Verification items for this drawing (mm, ordinates from the low corner). Coordinates: 2 decimals unless noted, no trailing zeros. Loops run counter-clockwise (first coordinate to the right, second up) from the corner with the lowest first, then second, coordinate; pieces in that order, holes last. Notation, with made-up numbers: M 36.5,27 L 40.5,27 A6 cw 40.5,35 Z; hole C -29,6.25 d4. An arc over 180 degrees is marked long. Write each question's results on one line, items separated by ' | '. Start each with the question number.
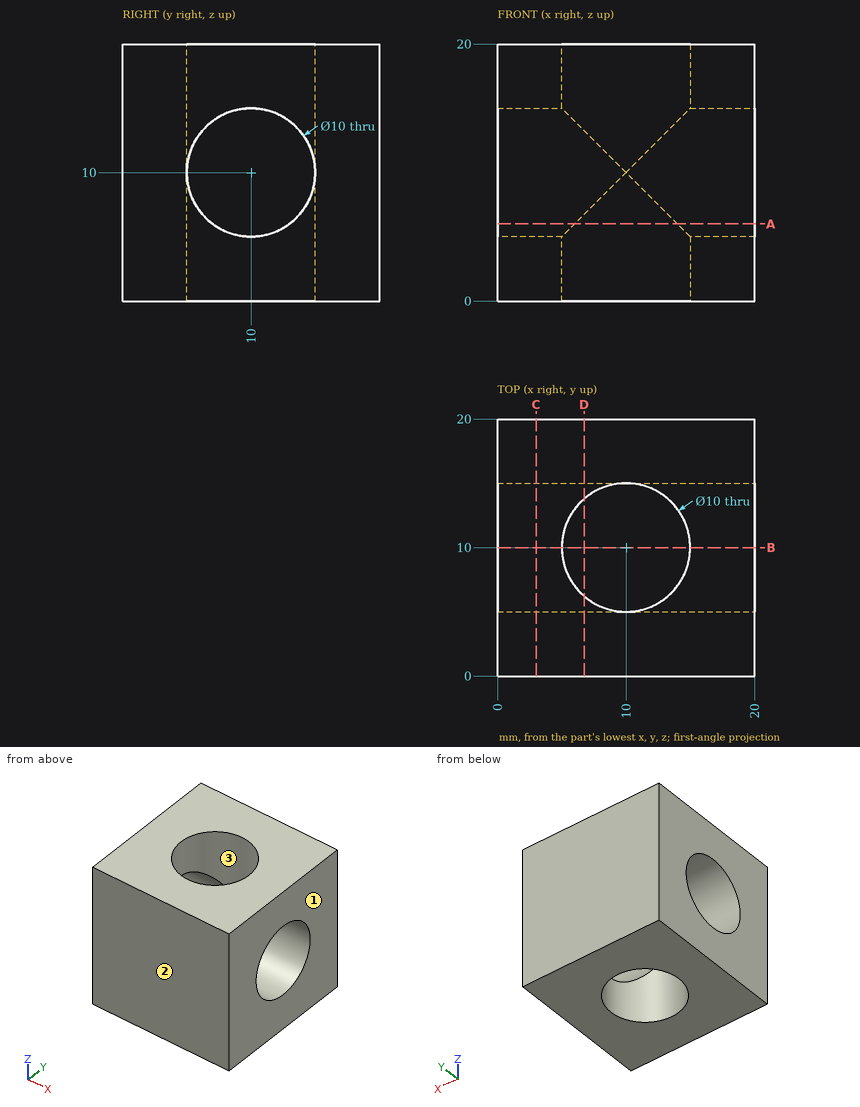
Item 1: Section check A-A (z = 6). Record the cut outline in (x, y).
Item 2: Release check for a two-part mould opening along X. For the marked faces 1, 2 and 3 record: +X half, -X half, draft (parallel to the pull), parting line (faces both ways), or undercut.
Item 3: Section check C-C (x = 3). Record the cut outline in (y, z).
Item 4: Depth check by flat-ended pin: P1, Ø10, axis at x = 13, z = 16.5, coming from the -Y side. Enter the tip coordinate at first touch or a pass-through.
Item 5: Section check D-D (x = 6.75). Record the cut outline in (y, z).
Item 6: Thickness scan on line 1 (Z direction, x = 4.5, y = 10). Record the ranges inside material, lowest first.
Item 7: Section check B-B (y = 10). Record the cut outline in (x, z), plus the area to 3 significant figures.
Computed values:
1) outline: M 0,0 L 20,0 L 20,7 L 14,7 A5 cw 6,7 L 0,7 Z; M 0,13 L 6,13 A5 cw 14,13 L 20,13 L 20,20 L 0,20 Z
2) face 1: +X half | face 2: draft | face 3: undercut
3) outline: M 0,0 L 20,0 L 20,20 L 0,20 Z; hole C 10,10 d10
4) P1: stops at y = 0
5) outline: M 0,0 L 6.2,0 L 6.2,6.75 A5 cw 6.2,13.25 L 6.2,20 L 0,20 Z; M 13.8,0 L 20,0 L 20,20 L 13.8,20 L 13.8,13.25 A5 cw 13.8,6.75 Z
6) line 1: z = 0 to 5, 15 to 20
7) outline: M 0,0 L 5,0 L 5,5 L 0,5 Z; M 0,15 L 5,15 L 5,20 L 0,20 Z; M 15,0 L 20,0 L 20,5 L 15,5 Z; M 15,15 L 20,15 L 20,20 L 15,20 Z | area: 100 mm²
